```python
from build123d import *

# Parameters (mm, degrees)
SKETCH1_R           = 30
BOSS_EXTRUDE1_DEPTH = 22
SKETCH2_R           = 10
CUT_EXTRUDE1_DEPTH  = 66
FILLET1_R           = 1
CUT_EXTRUDE2_DEPTH  = 2


with BuildPart() as part:
    # Sketch1 → Boss-Extrude1 (new body)
    with BuildSketch(Plane.XY):
        Circle(SKETCH1_R)
    extrude(amount=BOSS_EXTRUDE1_DEPTH)

    # Sketch2 → Cut-Extrude1 (cut)
    with BuildSketch(Plane(origin=(0, 0, 0), x_dir=(-1, 0, 0), z_dir=(0, 0, -1))):
        Circle(SKETCH2_R)
    extrude(amount=-CUT_EXTRUDE1_DEPTH, mode=Mode.SUBTRACT)

    # Fillet1
    fillet1_edges = [part.edges().sort_by_distance(p)[0] for p in [
        (-30, 0, 0),
        (-30, 0, 22),
    ]]
    fillet(fillet1_edges, radius=FILLET1_R)

    # Sketch3 → Cut-Extrude2 (cut)
    with BuildSketch(Plane(origin=(0, 0, 0), x_dir=(-1, 0, 0), z_dir=(0, 0, -1))):
        with BuildLine():
            Line((-0.5, 24.9949995), (-0.5, 3.464101615))
            ThreePointArc((-0.5, 3.464101615), (-2.474873734, 2.474873734), (-3.464101615, 0.5))
            Line((-3.464101615, 0.5), (-24.9949995, 0.5))
            ThreePointArc((-24.9949995, 0.5), (-17.67766953, 17.67766953), (-0.5, 24.9949995))
        make_face()
        with BuildLine():
            Line((0.5, 24.9949995), (0.5, 3.464101615))
            ThreePointArc((0.5, 3.464101615), (2.474873734, 2.474873734), (3.464101615, 0.5))
            Line((3.464101615, 0.5), (24.9949995, 0.5))
            ThreePointArc((24.9949995, 0.5), (17.67766953, 17.67766953), (0.5, 24.9949995))
        make_face()
        with BuildLine():
            Line((-24.9949995, -0.5), (-3.464101615, -0.5))
            ThreePointArc((-3.464101615, -0.5), (-2.474873734, -2.474873734), (-0.5, -3.464101615))
            Line((-0.5, -3.464101615), (-0.5, -24.9949995))
            ThreePointArc((-0.5, -24.9949995), (-17.67766953, -17.67766953), (-24.9949995, -0.5))
        make_face()
        with BuildLine():
            Line((0.5, -3.464101615), (0.5, -24.9949995))
            ThreePointArc((0.5, -24.9949995), (17.67766953, -17.67766953), (24.9949995, -0.5))
            Line((24.9949995, -0.5), (3.464101615, -0.5))
            ThreePointArc((3.464101615, -0.5), (2.474873734, -2.474873734), (0.5, -3.464101615))
        make_face()
    extrude(amount=-CUT_EXTRUDE2_DEPTH, mode=Mode.SUBTRACT)


solid = part.part
```
Can you work these out from the model? Positions are in its coordinate system, mm. A direction names the side the tool comes from. Round coordinates to 2 decimals unless told otherwise and drop trailing zeros. Order: outer loops, then holes, each group sorted by start corner. A loop starts at its lowest first (then second) coordinate and runs counter-clockwise, first axis right, second up.
(1) If I drill on L1, parallel to Y at x = 0, z = 14.5; L2, parallel to Z at x = -16.5, y = 8; L3, parallel to X at y = -1, z = 11.25, over which ranges is the centre line in solid material (lowest first)?
Results are:
L1: y = -30 to -10, 10 to 30
L2: z = 2 to 22
L3: x = -29.98 to -9.95, 9.95 to 29.98
(2) I'm going to push flat-ended pins straight in: pin 1 (2 mm diameter, centred on x = -16.5, z = 0.5, fed in from +Y); pin 2 (12 mm diameter, centred on y = 6.5, z = 9.5, fed in from +X); pin 3 (4 mm diameter, centred on y = 16.5, z = 9, fed in from -X). Where does each tip first touch, or does it pass through?
Results are:
pin 1: stops at y = 25.63
pin 2: stops at x = 30
pin 3: stops at x = -26.26
(3) We'd pull the mould along Y, two halves only. Please class faces 1 (the face through (12, 0, 22)), 2 (the face through (10, 0, 11)), 3 (the face through (-29.97, 1.32, 10.86)): +Y half, -Y half, draft (parallel to the pull), parting line (faces both ways), or undercut.
Results are:
face 1: draft
face 2: undercut
face 3: parting line
(4) If we section it at A-A (z = 13.5): Please give me the cut outline in (x, y).
Results are:
outline: circle Ø60 at (0, 0); hole circle Ø20 at (0, 0)
(5) On a 3-axis mill with a long thin cutter (end or side, diameter ignored), from which of +Z, -Z, +X, -X, +Y, -Y can I reach the whole of each face in a straight line? I mean faces 4 (the face through (-13, -13, 2)), 5 (the face through (0, 11, 0)). Say none if no direction works.
Results are:
face 4: -Z
face 5: -Z, +X, -X, +Y, -Y
